Read the model definition and answer for the solid it produces. Units are mm, in the model's axes. Face numbers are marked on the shaded views. A direction names the side the tool comes from. Coordinates: 2 decimals unless noted, no trailing zeros. Write each loop counter-clockwise with the first axis right and the second up, starting at its lowest first coordinate (ties: lowest second). Pieces come first, ordered by that corner, then holes.
from build123d import *

# Parameters (mm, degrees)
SKETCH_R      = 23.521413
SKETCH_R_2    = 17.427543
PAD_DEPTH     = 50
SKETCH001_R   = 42.802844
SKETCH001_R_2 = 11.661281
PAD001_DEPTH  = 20
SKETCH002_W   = 14
SKETCH002_H   = 29
PAD002_DEPTH  = 20


with BuildPart() as part:
    # Sketch → Pad (new body)
    with BuildSketch(Plane.XY):
        Circle(SKETCH_R)
        Circle(SKETCH_R_2, mode=Mode.SUBTRACT)
    extrude(amount=PAD_DEPTH)

    # Sketch001 → Pad001 (new body)
    with BuildSketch(Plane.XY.offset(50)):
        Circle(SKETCH001_R)
        Circle(SKETCH001_R_2, mode=Mode.SUBTRACT)
    extrude(amount=PAD001_DEPTH)

    # Sketch002 → Pad002 (new body)
    with BuildSketch(Plane.XY.offset(70)):
        with Locations((-29, 0)):
            Rectangle(SKETCH002_W, SKETCH002_H)
        with Locations((29, 0)):
            Rectangle(SKETCH002_W, SKETCH002_H)
    extrude(amount=PAD002_DEPTH)


solid = part.part
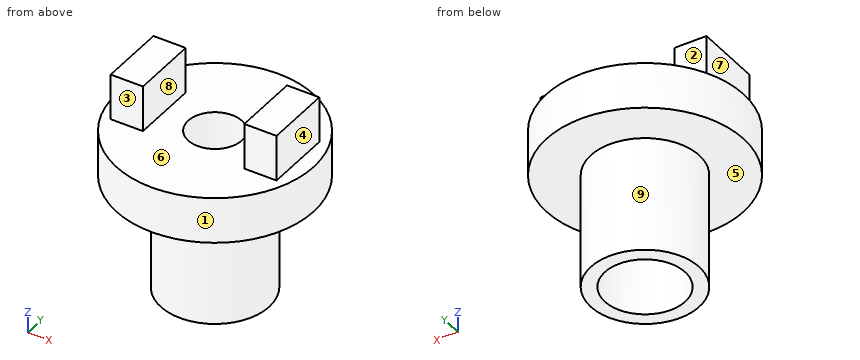
Item 1: Find the intervals of material crossed by probe 1 along Y at (x, z) = (0, 55.5); probe 2 along Y at (x, z) = (0, 21); probe 3 along Z at (x, y) = (-30, 0.5), in increasing order.
Item 2: The part is cut by section A-A (y = 0). Give the vertices of the cut face in (x, z).
Item 3: Given pin 1 (7 mm diameter, centred on x = -29.5, z = 81, fed in from -Y); pin 2 (10 mm diameter, centred on y = -7, z = 84.5, fed in from +X); pin 3 (3 mm diameter, centred on x = -8, y = 4, fed in from -Z); pin 4 (12 mm diameter, centred on x = -32.5, y = -21, fed in from +Z), each flat-ended and moving along its own axis, determine where each tip first touches the part or whether it passes through.
Item 4: The part is cut by section B-B (x = -3). Give the vertices of the cut face in (y, z), and give its area (3 significant figures).
Item 5: Determine the mould class of the marked faces 6, 7, 8 and 9 for opening direction X: +X half, -X half, draft (parallel to the pull), parting line (faces both ways), or undercut.
Item 6: For the marked faces 1, 2, 3, 4 and 5, determine the directions among +Z, -Z, +X, -X, +Y, -Y from which every point of the face is accessible in a straight line to the end or side of a thin tool.
Item 7: The part is cut by section C-C (z = 30). Give the vertices of the cut face in (x, y).
Item 8: The part is cut by section D-D (x = -31). Give the vertices of the cut face in (y, z), and give its area (3 significant figures).
Answer:
1. probe 1: y = -42.8 to -11.66, 11.66 to 42.8
1. probe 2: y = -23.52 to -17.43, 17.43 to 23.52
1. probe 3: z = 50 to 90
2. outline: (-42.8, 50) - (-23.52, 50) - (-23.52, 0) - (-17.43, 0) - (-17.43, 50) - (-11.66, 50) - (-11.66, 70) - (-22, 70) - (-22, 90) - (-36, 90) - (-36, 70) - (-42.8, 70) - close; (11.66, 50) - (17.43, 50) - (17.43, 0) - (23.52, 0) - (23.52, 50) - (42.8, 50) - (42.8, 70) - (36, 70) - (36, 90) - (22, 90) - (22, 70) - (11.66, 70) - close
3. pin 1: stops at y = -14.5
3. pin 2: stops at x = 36
3. pin 3: passes through
3. pin 4: stops at z = 70
4. outline: (-42.7, 50) - (-23.33, 50) - (-23.33, 0) - (-17.17, 0) - (-17.17, 50) - (-11.27, 50) - (-11.27, 70) - (-42.7, 70) - close; (11.27, 50) - (17.17, 50) - (17.17, 0) - (23.33, 0) - (23.33, 50) - (42.7, 50) - (42.7, 70) - (11.27, 70) - close
4. area: 1,870 mm2
5. face 6: undercut
5. face 7: -X half
5. face 8: undercut
5. face 9: parting line
6. face 1: +Z, -Z
6. face 2: +Z, +X, -X, +Y
6. face 3: +Z, +X, -X, -Y
6. face 4: +Z, +X, +Y, -Y
6. face 5: -Z
7. outline: circle Ø47.04 at (0, 0); hole circle Ø34.86 at (0, 0)
8. outline: (-29.51, 50) - (29.51, 50) - (29.51, 70) - (14.5, 70) - (14.5, 90) - (-14.5, 90) - (-14.5, 70) - (-29.51, 70) - close
8. area: 1,760 mm2
